Design review of the part built by this model. Coordinates are the model's own, in mm. Face numbers are marked on the shaded views. Give positions to 0.01 mm unless a question says otherwise; leave off trailing zeros. Loops run counter-clockwise (first coordinate to the right, second up) from the corner with the lowest first, then second, coordinate; pieces in that order, holes last. Notation, with made-up numbers: (18.25, 30) - (52.25, 30) arc R18 cw to (52.25, 49) - close; hole circle Ø2 at (-17, 29). An arc over 180 degrees is marked (long way). Write each question's results on one line, items separated by ' | '.
```python
from build123d import *

# Parameters (mm, degrees)
SKETCH1_W           = 125
SKETCH1_H           = 300
SKETCH1_R           = 5
BOSS_EXTRUDE1_DEPTH = 5
SKETCH2_R           = 30
BOSS_EXTRUDE2_DEPTH = 800
SKETCH3_R           = 30
BOSS_EXTRUDE3_DEPTH = 225


with BuildPart() as part:
    # Sketch1 → Boss-Extrude1 (new body)
    with BuildSketch(Plane(origin=(0, 0, 0), x_dir=(1, 0, 0), z_dir=(0, 1, 0))):
        Rectangle(SKETCH1_W, SKETCH1_H)
        with Locations(Location((-47.5, 135, 0), (0, 0, 270))):
            Circle(SKETCH1_R, mode=Mode.SUBTRACT)
        with Locations(Location((47.5, -135, 0), (0, 0, 270))):
            Circle(SKETCH1_R, mode=Mode.SUBTRACT)
        with BuildLine():
            Line((-47.5, 50), (-37.5, 50))
            ThreePointArc((-37.5, 50), (-32.5, 45), (-37.5, 40))
            Line((-37.5, 40), (-47.5, 40))
            ThreePointArc((-47.5, 40), (-52.5, 45), (-47.5, 50))
        make_face(mode=Mode.SUBTRACT)
        with BuildLine():
            Line((-47.5, -40), (-37.5, -40))
            ThreePointArc((-37.5, -40), (-32.5, -45), (-37.5, -50))
            Line((-37.5, -50), (-47.5, -50))
            ThreePointArc((-47.5, -50), (-52.5, -45), (-47.5, -40))
        make_face(mode=Mode.SUBTRACT)
        with BuildLine():
            Line((-47.5, -130), (-37.5, -130))
            ThreePointArc((-37.5, -130), (-32.5, -135), (-37.5, -140))
            Line((-37.5, -140), (-47.5, -140))
            ThreePointArc((-47.5, -140), (-52.5, -135), (-47.5, -130))
        make_face(mode=Mode.SUBTRACT)
        with BuildLine():
            Line((47.5, -50), (37.5, -50))
            ThreePointArc((37.5, -50), (32.5, -45), (37.5, -40))
            Line((37.5, -40), (47.5, -40))
            ThreePointArc((47.5, -40), (52.5, -45), (47.5, -50))
        make_face(mode=Mode.SUBTRACT)
        with BuildLine():
            Line((47.5, 40), (37.5, 40))
            ThreePointArc((37.5, 40), (32.5, 45), (37.5, 50))
            Line((37.5, 50), (47.5, 50))
            ThreePointArc((47.5, 50), (52.5, 45), (47.5, 40))
        make_face(mode=Mode.SUBTRACT)
        with BuildLine():
            Line((47.5, 130), (37.5, 130))
            ThreePointArc((37.5, 130), (32.5, 135), (37.5, 140))
            Line((37.5, 140), (47.5, 140))
            ThreePointArc((47.5, 140), (52.5, 135), (47.5, 130))
        make_face(mode=Mode.SUBTRACT)
    extrude(amount=-BOSS_EXTRUDE1_DEPTH)

    # Sketch2 → Boss-Extrude2 (add)
    with BuildSketch(Plane(origin=(0, -5, 0), x_dir=(-1, 0, 0), z_dir=(0, -1, 0))):
        with Locations(Location((0, 0, 0), (0, 0, 270))):
            Circle(SKETCH2_R)
    extrude(amount=BOSS_EXTRUDE2_DEPTH)

    # Sketch3 → Boss-Extrude3 (add, symmetric)
    with BuildSketch(Plane.XY):
        with Locations((0, -805)):
            Circle(SKETCH3_R)
    extrude(amount=BOSS_EXTRUDE3_DEPTH, both=True)


solid = part.part
```
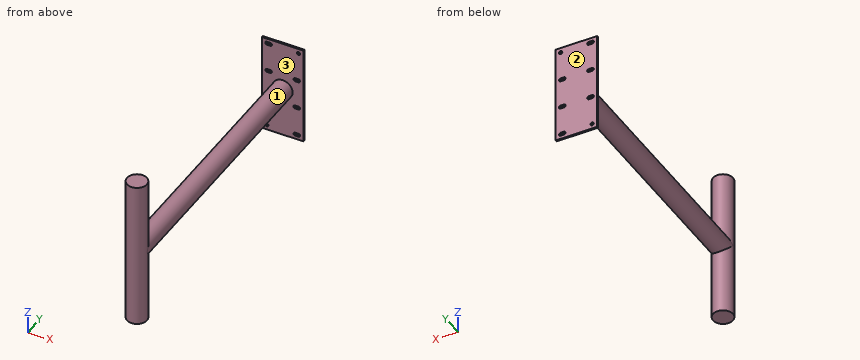
Item 1: We need section B-B on z = -11. Give the boundary of the cut face in (x, y).
Output values:
outline: (-62.5, -5) - (-27.91, -5) - (-27.91, -794) arc R30 ccw (long way) to (27.91, -794) - (27.91, -5) - (62.5, -5) - (62.5, 0) - (-62.5, 0) - close
Item 2: We need section A-A on z = -120. Give the boundary of the cut face in (x, y).
Output values:
outline: (-62.5, -5) - (62.5, -5) - (62.5, 0) - (-62.5, 0) - close; circle Ø60 at (0, -805)
Item 3: We need section C-C on y = -175. Give the boundary of the cut face in (x, z), then the cut area to 3 significant figures.
Output values:
outline: circle Ø60 at (0, 0) | area: 2,830 mm²
Item 4: Wall thickness on probe 1 along X at (y, z) = (-3.2, -135); probe 2 along X at (y, z) = (-2, 135); probe 3 along Y at (x, z) = (0.5, -43): over which ranges is each line inside the solid? List them lowest first.
Output values:
probe 1: x = -62.5 to -52.5, -42.5 to 32.5, 52.5 to 62.5 | probe 2: x = -62.5 to -52.5, -32.5 to 42.5, 52.5 to 62.5 | probe 3: y = -835 to -775, -5 to 0
Item 5: Draft analysis for pull direction Y (two halves, no side actions). For the marked faces 1, 2 and 3, state which applies: +Y half, -Y half, draft (parallel to the pull), parting line (faces both ways), or undercut.
Output values:
face 1: undercut | face 2: +Y half | face 3: undercut
Item 6: Clearance check with flat-ended pins moving along their axes: P1, Ø2.5, axis at x = -43.5, y = -2, coming from the -Z side; P2, Ø13, axis at x = -47.5, z = -135, coming from the -Y side; P3, Ø4, axis at x = -43, y = -3, coming from the +Z side; P4, Ø16, axis at x = 47.5, z = 135, coming from the +Y side. State where each tip first meets the part, or that it passes through.
Output values:
P1: stops at z = -150 | P2: stops at y = -5 | P3: stops at z = 150 | P4: stops at y = 0
